Work out the finished part from the listing and answer in its coordinate system (mm). A direction names the side the tool comes from. Give positions to 0.01 mm unless a question says otherwise; leave off trailing zeros. Order: outer loops, then holes, each group sorted by start corner. A loop starts at its lowest first (then second) coordinate and runs counter-clockwise, first axis right, second up.
```python
from build123d import *

# Parameters (mm, degrees)
BOSS_EXTRUDE1_DEPTH      = 3.5
BOSS_EXTRUDE1_DEPTH_BACK = 3.5
SKETCH1_R                = 1.6
CUT_EXTRUDE1_REACH       = 28.632
SKETCH3_R                = 1.6
SKETCH3_3_R              = 2.2
SKETCH3_3_R_2            = 1.6
CUT_EXTRUDE2_DEPTH       = 6
CUT_EXTRUDE3_REACH       = 28.632
FILLET1_R                = 2
FILLET2_R                = 0.4


with BuildPart() as part:
    # Sketch1 → Boss-Extrude1 (new, two sides: drawn at the far end of the back side and taken through both)
    with BuildSketch(Plane.XY.offset(-BOSS_EXTRUDE1_DEPTH_BACK)):
        with BuildLine():
            Line((-21, 8), (-18.64966284, 8))
            Line((-18.64966284, 8), (-10, -0.5))
            Line((-10, -0.5), (-3.979949748, -0.4))
            ThreePointArc((-3.979949748, -0.4), (0, -4), (3.979949748, -0.4))
            Line((3.979949748, -0.4), (6, -0.4))
            Line((6, -0.4), (6, 0.4))
            Line((6, 0.4), (3.979949748, 0.4))
            ThreePointArc((3.979949748, 0.4), (0, 4), (-3.979949748, 0.4))
            Line((-3.979949748, 0.4), (-10, 0.5))
            Line((-10, 0.5), (-16.848441102, 8))
            Line((-16.848441102, 8), (21, 8))
            Line((21, 8), (21, -8))
            Line((21, -8), (-21, -8))
            Line((-21, -8), (-21, 8))
        make_face()
        with Locations((-18, 0)):
            Circle(SKETCH1_R, mode=Mode.SUBTRACT)
        with Locations(Location((18, 0, 0), (0, 0, 180))):
            Circle(SKETCH1_R, mode=Mode.SUBTRACT)
    extrude(amount=BOSS_EXTRUDE1_DEPTH + BOSS_EXTRUDE1_DEPTH_BACK)

    # Cut-Extrude1: up to this plane
    cut_extrude1_end = Plane(origin=(-10, -0.5, -3.5), z_dir=(-0.016608865731892127, 0.9998620632762801, 0))
    # Sketch3 → Cut-Extrude1 (cut, up to the surface)
    with BuildSketch(Plane.XZ.offset(8), mode=Mode.PRIVATE) as cut_extrude1_sk1:
        with Locations(Location((-6.989974874, 0, 0), (0, 0, 270))):
            Circle(SKETCH3_R)
    cut_extrude1_tool1 = split(extrude(cut_extrude1_sk1.sketch, amount=-CUT_EXTRUDE1_REACH, mode=Mode.PRIVATE), bisect_by=cut_extrude1_end, keep=Keep.BOTH, mode=Mode.PRIVATE)
    add(cut_extrude1_tool1.solids().sort_by_distance((-6.989975, -8, 0))[0], mode=Mode.SUBTRACT)

    # Sketch3<3> → Cut-Extrude2 (cut)
    with BuildSketch(Plane.XZ.offset(8)):
        with Locations(Location((-6.989974874, 0, 0), (0, 0, 270))):
            Circle(SKETCH3_3_R)
        with Locations(Location((-6.989974874, 0, 0), (0, 0, 270))):
            Circle(SKETCH3_3_R_2, mode=Mode.SUBTRACT)
    extrude(amount=-CUT_EXTRUDE2_DEPTH, mode=Mode.SUBTRACT)

    # Cut-Extrude3: up to this plane
    cut_extrude3_end = Plane(origin=(-10, 0.5, -3.5), z_dir=(-0.016608865731892127, -0.9998620632762801, 0))
    # Sketch4 → Cut-Extrude3 (cut, up to the surface)
    with BuildSketch(Plane(origin=(0, 8, 0), x_dir=(1, 0, 0), z_dir=(0, 1, 0)), mode=Mode.PRIVATE) as cut_extrude3_sk1:
        with BuildLine():
            Line((-7.489974874, 1.6), (-6.489974874, 1.6))
            ThreePointArc((-6.489974874, 1.6), (-4.889974874, 0), (-6.489974874, -1.6))
            Line((-6.489974874, -1.6), (-7.489974874, -1.6))
            ThreePointArc((-7.489974874, -1.6), (-9.089974874, 0), (-7.489974874, 1.6))
        make_face()
    cut_extrude3_tool1 = split(extrude(cut_extrude3_sk1.sketch, amount=-CUT_EXTRUDE3_REACH, mode=Mode.PRIVATE), bisect_by=cut_extrude3_end, keep=Keep.BOTH, mode=Mode.PRIVATE)
    add(cut_extrude3_tool1.solids().sort_by_distance((-6.989975, 8, 0))[0], mode=Mode.SUBTRACT)

    # Fillet1
    fillet1_edges = [part.edges().sort_by_distance(p)[0] for p in [
        (21, 8, 0),
        (21, -8, 0),
        (-21, -8, 0),
        (-21, 8, 0),
    ]]
    fillet(fillet1_edges, radius=FILLET1_R)

    # Fillet2
    fillet2_edges = [part.edges().sort_by_distance(p)[0] for p in [
        (6, -0.4, 0),
        (6, 0.4, 0),
    ]]
    fillet(fillet2_edges, radius=FILLET2_R - 0.0001)  # a hair under: the kernel refuses the full size


solid = part.part
```
1. The mould has two halves that part along Y. Classify faces 4 (the face through (-9, -2, 0)), 5 (the face through (-13.38, 4.2, -0.05)), 6 (the face through (-20.4, 7.43, 0.05)), 7 (the face through (-9.138, -5.042, 0.477)): pulls with the +Y half, pulls with the -Y half, needs draft (parallel to the pull), parting line crosses it, or undercut.
Findings below:
face 4: pulls with the -Y half
face 5: undercut
face 6: pulls with the +Y half
face 7: needs draft
2. The part is cut by section A-A (x = 18). Write down the section's boundary in (y, z).
Findings below:
outline: (-8, -3.5) - (-1.6, -3.5) - (-1.6, 3.5) - (-8, 3.5) - close; (1.6, -3.5) - (8, -3.5) - (8, 3.5) - (1.6, 3.5) - close
3. The part is cut by section C-C (y = -3.25). Write down the section's boundary in (x, z).
Findings below:
outline: (-21, -3.5) - (-2.33, -3.5) - (-2.33, 3.5) - (-21, 3.5) - close; (2.33, -3.5) - (21, -3.5) - (21, 3.5) - (2.33, 3.5) - close; hole circle Ø4.4 at (-6.99, 0)
4. The part is cut by section B-B (z = 0). State how many separate pieces and enclosed holes the cut face has, then the cut area to 3 significant figures.
Findings below:
separate pieces: 3
enclosed holes: 2
area: 521 mm2
5. Given P1, Ø2.5, axis at x = 18, y = 0, coming from the -Z side; P2, Ø4, axis at x = -6.99, z = 0, coming from the -Y side, each flat-ended and moving along its own axis, determine where each tip first touches the part or whether it passes through.
Findings below:
P1: passes through
P2: stops at y = -2
6. Which of the six approach directions +Z, -Z, +X, -X, +Y, -Y give full straight-line access (tool end or side, diameter ignored) to faces 1 (the face through (1, 8, 0)), 2 (the face through (-9.09, 4.28, 0.04)), 3 (the face through (0, 4, 0))?
Findings below:
face 1: +Z, -Z, +X, -X, +Y
face 2: +Y
face 3: +Z, -Z
7. Straight lines are drawn through the part: probe 1 along X at (y, z) = (-0.7, 0); probe 2 along X at (y, z) = (2, 1.25); probe 3 along X at (y, z) = (-1.45, 0). For each, find the intervals that lie inside material, in ascending order.
Findings below:
probe 1: x = -21 to -19.44, -16.56 to -8.59, -5.39 to -3.94, 3.94 to 16.56, 19.44 to 21
probe 2: x = -21 to -12.54, -11.37 to -8.49, -5.49 to -3.46, 3.46 to 21
probe 3: x = -21 to -18.68, -17.32 to -8.59, -5.39 to -3.73, 3.73 to 17.32, 18.68 to 21
